Geometry: final body of the model. Coordinates: model frame, mm. A direction names the side the tool comes from. Round coordinates to 2 decimals unless told otherwise and drop trailing zeros. Loops run counter-clockwise (first coordinate to the right, second up) from the corner with the lowest first, then second, coordinate; pieces in that order, holes last. Notation, with made-up numbers: (74, 80) - (84, 80) arc R38 ccw to (84, 119) - close; hole circle Ø1 at (34.25, -18). An arc over 180 degrees is marked (long way). Answer as CSV lines item,"result".
Autodesk Inventor part; units mm, degrees
ref_plane "YZ Plane" through (0, 0, 0) normal (1, 0, 0) x (0, 1, 0)
ref_plane "XZ Plane" through (0, 0, 0) normal (0, 1, 0) x (-1, 0, 0)
ref_plane "XY Plane" through (0, 0, 0) normal (0, 0, 1) x (1, 0, 0)
sketch "Skizze1" plane through (0, 0, 0) normal (1, 0, 0) x (0, 1, 0)
  line L0 (25.8, 0) -> (20.8, 0)
  line L1 (20.8, 0) -> (20.8, -10)
  line L2 (20.8, -10) -> (25.8, -10)
  line L3 (25.8, -10) -> (25.8, 0)
  line L4 (18, -57.6) -> (12, -57.6)
  line L5 (12, -57.6) -> (12, -47.6)
  line L6 (12, -47.6) -> (18, -47.6)
  line L7 (18, -47.6) -> (18, -57.6)
  line L8 (25.8, -10) -> (18, -47.6)
  line L9 (20.8, -10) -> (12, -47.6)
  line L10 (12, -57.6) -> (15, -57.6)
  line L11 (15, -57.6) -> (15, -52.6)
  line L12 (15, -52.6) -> (12, -52.6)
  line L13 (12, -52.6) -> (12, -57.6)
  line L14 (0, -70.72) -> (0, 21.12)
  line L15 (25.8, 0) -> (20.8, 0)
  line L16 (20.8, 0) -> (20.8, 8)
  line L17 (20.8, 8) -> (25.8, 8)
  line L18 (25.8, 8) -> (25.8, 0)
  line L19 (25.8, 0) -> (26.8, 0)
  line L20 (26.8, 0) -> (26.8, -3)
  line L21 (26.8, -3) -> (25.8, -3)
  line L22 (25.8, -3) -> (25.8, 0)
  line L23 (26.8, -3) -> (25.8, -5.6618)
  point P0 (0, 0)
  point P1 (15, -57.6)
  point P2 (15, -47.6)
  point P3 (15, -55.1)
  dimension "d0" = 5
  dimension "d1" = 10
  dimension "d2" = 25.8
  dimension "d3" = 57.6
  dimension "d4" = 10
  dimension "d5" = 6
  dimension "d6" = 12
  dimension "d7" = 5
  dimension "d8" = 15
  dimension "d16" = 8
  dimension "d17" = 1
  dimension "d18" = 3
revolve "Umdrehung1" add sketch "Skizze1" angle 360 about axis through (0, 0, -10) along (0, 0, 1) contours L3 L2 L1 L0 | L19 L20 L21 L3 | L0 L16 L17 L18 | L21 L23 L3 | L2 L8 L6 L9 | L6 L7 L4 L11 L12 L5
sketch "Skizze2" plane through (0, 0, 0) normal (0, 1, 0) x (-1, 0, 0)
  circle A0 centre (0, -55.252) radius 1.4
  point P0 (0, 0)
  dimension "d10" = 2.8
extrude "Extrusion1" cut sketch "Skizze2" against normal through all
pattern_circular "Runde Anordnung1" count 3 over 360 about axis through (0, 0, -52.6) along (0, 0, 1) of "Extrusion1"
properties part number "00_Zeiss_Daheng_Adapter"
(1) Pin query (flat end, axial travel): P1, Ø2, axis at x = 0, z = -55.252, coming from the -Y side; P2, Ø1, axis at y = 8.5, z = -17, coming from the +X side; P3, Ø5, axis at y = -9, z = -39, coming from the -X side. Return the tip coordinate at first contact, or that it passes through.
Findings below:
P1,"y = 14.97"
P2,"x = 23.03"
P3,"x = -18.84"
(2) Section A-A (y = 0). Output: boundary loops of the cut face in (x, z).
Findings below:
outline,"(-26.8, -3) - (-25.8, -5.66) - (-25.8, -10) - (-18, -47.6) - (-18, -57.6) - (-15, -57.6) - (-15, -52.6) - (-12, -52.6) - (-12, -47.6) - (-20.8, -10) - (-20.8, 8) - (-25.8, 8) - (-25.8, 0) - (-26.8, 0) - close; (12, -52.6) - (15, -52.6) - (15, -57.6) - (18, -57.6) - (18, -47.6) - (25.8, -10) - (25.8, -5.66) - (26.8, -3) - (26.8, 0) - (25.8, 0) - (25.8, 8) - (20.8, 8) - (20.8, -10) - (12, -47.6) - close"
(3) Access query for faces 5 (the face through (-14, -22, 0)), 6 (the face through (-0.53, -11.99, -50.06)), 7 (the face through (-10, -7, -52.6)). Directions: +Z, -Z, +X, -X, +Y, -Y. A direction counts if a zero-diameter tool reaches every point of the face in a straight line with its end or side. Return the directions, or none.
Findings below:
face 5,"+Z"
face 6,"+Z, -Z"
face 7,"-Z"
(4) Section C-C (z = -15.5). Output: boundary loops of the cut face in (x, y), and give its area (3 significant figures).
Findings below:
outline,"circle Ø49.32 at (0, 0); hole circle Ø39.03 at (0, 0)"
area,"714 mm2"
(5) Section B-B (x = 0). Give the number of separate pieces and of enclosed holes in the cut face, and give its area (3 significant figures).
Findings below:
separate pieces,"3"
enclosed holes,"0"
area,"684 mm2"
(6) Section D-D (z = -46.5). Output: boundary loops of the cut face in (x, y).
Findings below:
outline,"circle Ø36.46 at (0, 0); hole circle Ø24.51 at (0, 0)"
(7) Material intervals for line 1 along Y through (x, z) = (0, -51); line 2 along Y through (x, z) = (0, 2.5); line 3 along X through (y, z) = (0, -55.55), sorted ascending.
Findings below:
line 1,"-18 to -12, 12 to 18"
line 2,"-25.8 to -20.8, 20.8 to 25.8"
line 3,"-18 to -15, 15 to 18"
(8) Draft query along Z for faces 1 (the face through (14.151, 8.381, -53.864)), 2 (the face through (0.182, -16.446, -53.864)), 3 (the face through (-20.91, -2.75, -32.71)), 4 (the face through (-20.623, -2.708, -0.874)). Return one class per face: pulls with the +Z half, pulls with the -Z half, needs draft (parallel to the pull), parting line crosses it, or undercut.
Findings below:
face 1,"undercut"
face 2,"undercut"
face 3,"pulls with the -Z half"
face 4,"needs draft"
